Input: part model. Units: mm. Frame: model coordinates. Face numbers are marked on the shaded views. A direction names the side the tool comes from. Give positions to 0.01 mm unless a question says otherwise; leave off trailing zeros. Order: outer loops, then holes, each group sorted by start corner. A loop starts at its lowest first (then second) coordinate and runs counter-clockwise, first axis right, second up. Notation, with made-up numbers: (54, 46.25) - (58, 46.25) arc R7 cw to (58, 53.25) - close; hole circle Ø10 at (-17.75, 45). An arc over 180 degrees is marked (long way). Answer in a Markdown table with one row per item. Add a question column.
1. Access query for the marked faces 4, 5 and 6. Directions: +Z, -Z, +X, -X, +Y, -Y. A direction counts if a zero-diameter tool reaches every point of the face in a straight line with its end or side. Return the directions, or none.
2. Section query C-C on z = 1.25. Return loops of the section in (x, y).
3. Ray query, line 1 (Y direction, x = 6.75, z = 1.25); line 2 (Y direction, x = 16.75, z = -1.75); line 3 (Z direction, x = 7.5, y = 4.25) (1 decimal). Return the intervals inside material, ascending. Write a range as [from, to].
4. Section query B-B on y = -1.25. Return loops of the section in (x, z) (1 decimal).
5. Section query A-A on x = 11.25. Return loops of the section in (y, z) (1 decimal).
6. Mould query, pull axis X, two halves, no side actions, for the marked faces 1, 2 and 3. Classes: released by +X, released by -X, zero draft, split by the parting line, or undercut.
7. Section query D-D on y = 4.5. Return loops of the section in (x, z) (1 decimal).
8. Contact query for flat-ended pins moving along their axis: pin 1 (0.8 mm diameter, centred on y = 3, z = -2, fed in from -X); pin 2 (3 mm diameter, centred on y = 4.5, z = 1.5, fed in from -X); pin 3 (2.5 mm diameter, centred on x = 10.5, z = 2.5, fed in from +Y); pin 4 (0.5 mm diameter, centred on y = 6, z = -2.5, fed in from +X). Output: stop coordinate, or through.
```python
from build123d import *

# Parameters (mm, degrees)
SKETCH1_W           = 1.5875
SKETCH1_H           = 1.5875
BOSS_EXTRUDE1_DEPTH = 4.8514
SKETCH2_W           = 28.575
SKETCH2_H           = 4.8514
BOSS_EXTRUDE2_DEPTH = 3.175
SKETCH3_W           = 6.35
SKETCH3_H           = 1.5875
BOSS_EXTRUDE3_DEPTH = 6.35
SKETCH4_R           = 2.286
CUT_EXTRUDE1_DEPTH  = 6.35


with BuildPart() as part:
    # Sketch1 → Boss-Extrude1 (new body)
    with BuildSketch(Plane.XY):
        Polygon((0, 1.5875), (0, 0), (25.4, 0), (25.4, -1.6764), (26.9875, -1.6764), (26.9875, 1.5875), align=None)
        with Locations((-0.79375, 0.79375)):
            Rectangle(SKETCH1_W, SKETCH1_H)
        Polygon((0, -1.6764), (0, 0), (-1.5875, 0), (-1.5875, -3.2639), (25.4, -3.2639), (25.4, -1.6764), align=None)
        with Locations((26.19375, -2.47015)):
            Rectangle(SKETCH1_W, SKETCH1_H)
    extrude(amount=BOSS_EXTRUDE1_DEPTH)

    # Sketch2 → Boss-Extrude2 (add)
    with BuildSketch(Plane(origin=(0, 0, 0), x_dir=(-1, 0, 0), z_dir=(0, 0, -1))):
        with Locations((-12.7, -0.8382)):
            Rectangle(SKETCH2_W, SKETCH2_H)
    extrude(amount=BOSS_EXTRUDE2_DEPTH)

    # Sketch3 → Boss-Extrude3 (add)
    with BuildSketch(Plane(origin=(0, 1.5875, 0), x_dir=(1, 0, 0), z_dir=(0, 1, 0))):
        with Locations((16.80095606, 2.38125)):
            Rectangle(SKETCH3_W, SKETCH3_H)
        Polygon((13.62595606, 3.175), (12.7, 3.175), (7.27595606, 3.175), (7.27595606, 1.5875), (13.62595606, 1.5875), align=None)
    extrude(amount=BOSS_EXTRUDE3_DEPTH)

    # Sketch4 → Cut-Extrude1 (cut)
    with BuildSketch(Plane.XY.offset(-1.5875)):
        with BuildLine():
            ThreePointArc((19.08695606, 4.7625), (16.80095606, 7.0485), (14.51495606, 4.7625))
            Line((14.51495606, 4.7625), (19.08695606, 4.7625))
        make_face()
        with BuildLine():
            Line((19.08695606, 4.7625), (14.51495606, 4.7625))
            ThreePointArc((14.51495606, 4.7625), (16.80095606, 2.4765), (19.08695606, 4.7625))
        make_face()
        with Locations((10.45095606, 4.7625)):
            Circle(SKETCH4_R)
    extrude(amount=-CUT_EXTRUDE1_DEPTH, mode=Mode.SUBTRACT)


solid = part.part
```
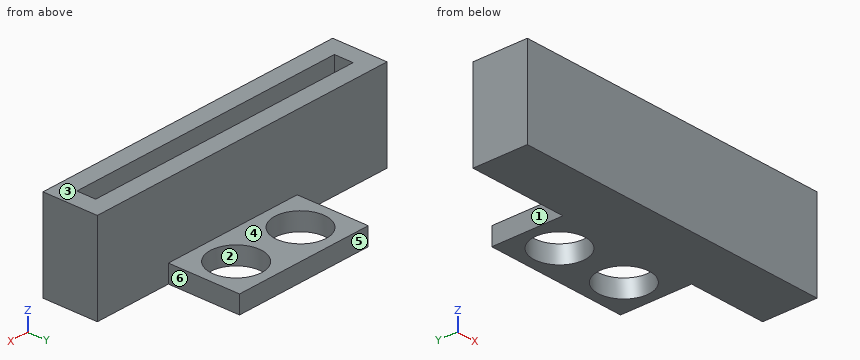
Answer:
| question | item | result |
|---|---|---|
| 1 | face 4 | +Z, +X, -X, +Y |
| 1 | face 5 | +Z, -Z, +X, -X, +Y |
| 1 | face 6 | +Z, -Z, +X, +Y |
| 2 | outline | (-1.59, -3.26) - (26.99, -3.26) - (26.99, 1.59) - (-1.59, 1.59) - close; hole (0, -1.68) - (25.4, -1.68) - (25.4, 0) - (0, 0) - close |
| 3 | line 1 | y = [-3.26, -1.68], [0, 1.59] |
| 3 | line 2 | y = [-3.26, 2.48], [7.05, 7.94] |
| 3 | line 3 | z = [-3.2, -1.6] |
| 4 | outline | (-1.6, -3.2) - (27, -3.2) - (27, 4.9) - (25.4, 4.9) - (25.4, 0) - (0, 0) - (0, 4.9) - (-1.6, 4.9) - close |
| 5 | outline | (-3.3, -3.2) - (2.6, -3.2) - (2.6, -1.6) - (1.6, -1.6) - (1.6, 4.9) - (0, 4.9) - (0, 0) - (-1.7, 0) - (-1.7, 4.9) - (-3.3, 4.9) - close; (6.9, -3.2) - (7.9, -3.2) - (7.9, -1.6) - (6.9, -1.6) - close |
| 6 | face 1 | released by -X |
| 6 | face 2 | undercut |
| 6 | face 3 | zero draft |
| 7 | outline | (7.3, -3.2) - (8.2, -3.2) - (8.2, -1.6) - (7.3, -1.6) - close; (12.7, -3.2) - (14.5, -3.2) - (14.5, -1.6) - (12.7, -1.6) - close; (19.1, -3.2) - (20, -3.2) - (20, -1.6) - (19.1, -1.6) - close |
| 8 | pin 1 | stops at x = 7.28 |
| 8 | pin 2 | passes through |
| 8 | pin 3 | stops at y = 1.59 |
| 8 | pin 4 | stops at x = 19.98 |
